from build123d import *

# Parameters (mm, degrees)
SKETCH1_R           = 237
SKETCH1_R_2         = 225
BOSS_EXTRUDE1_DEPTH = 2
SKETCH2_R           = 227
SKETCH2_R_2         = 225
EXTRUDE_THIN1_DEPTH = 50
SKETCH3_R           = 237
SKETCH3_R_2         = 225
EXTRUDE_THIN2_DEPTH = 2


with BuildPart() as part:
    # Sketch1 → Boss-Extrude1 (new body)
    with BuildSketch(Plane(origin=(0, 0, 0), x_dir=(1, 0, 0), z_dir=(0, 1, 0))):
        with Locations(Location((0, 0, 0), (0, 0, 270))):
            Circle(SKETCH1_R)
        with Locations(Location((0, 0, 0), (0, 0, 270))):
            Circle(SKETCH1_R_2, mode=Mode.SUBTRACT)
    extrude(amount=BOSS_EXTRUDE1_DEPTH)

    # Sketch2 → Extrude-Thin1 (add)
    with BuildSketch(Plane(origin=(0, 2, 0), x_dir=(1, 0, 0), z_dir=(0, 1, 0))):
        Circle(SKETCH2_R)
        Circle(SKETCH2_R_2, mode=Mode.SUBTRACT)
    extrude(amount=EXTRUDE_THIN1_DEPTH)

    # Sketch3 → Extrude-Thin2 (add)
    with BuildSketch(Plane(origin=(0, 52, 0), x_dir=(1, 0, 0), z_dir=(0, 1, 0))):
        Circle(SKETCH3_R)
        Circle(SKETCH3_R_2, mode=Mode.SUBTRACT)
    extrude(amount=EXTRUDE_THIN2_DEPTH)


solid = part.part
Input: part model. Units: mm. Frame: model coordinates. A direction names the side the tool comes from. Give positions to 0.01 mm unless a question says otherwise; leave off trailing zeros. Loops run counter-clockwise (first coordinate to the right, second up) from the corner with the lowest first, then second, coordinate; pieces in that order, holes last. Notation, with made-up numbers: (82.25, -32.5) -> (108.25, -32.5) arc R14 ccw to (108.25, -22.5) -> close; hole circle Ø11 at (-25, 48). An arc over 180 degrees is marked (long way). Answer as a JSON object with one key per item and string values. Group by question number.
Item 1: Reachability of faces 1 (the flat face through (210, 54, 87)), 2 (the cylindrical face through (-167.308, 26.65, -153.417)) from +Z, -Z, +X, -X, +Y, -Y: full face, straight path, thin tool, end or side. Return the list, or none.
Item 2: Cut plane B-B, the plane z = -47. Return the cut outline in (x, y), and give its area (3 significant figures).
Item 3: Line query: probe 1 along X at (y, z) = (19, 0); probe 2 along Z at (x, y) = (66.5, 48). Output: solid intervals per line, ascending.
Item 4: Cut plane C-C, the plane y = 7.5. Return the cut outline in (x, z).
Item 5: Pin query (flat end, axial travel): P1, Ø12, axis at x = 128, y = 26.5, coming from the +Z side; P2, Ø1, axis at y = 28, z = -152, coming from the +X side; P3, Ø4, axis at y = 44, z = -22, coming from the -X side. Return the tip coordinate at first contact, or that it passes through.
Checks:
{
 "1": {"face 1": "+Z, -Z, +X, -X, +Y", "face 2": "none"},
 "2": {"outline": "(-232.29, 0) -> (-220.04, 0) -> (-220.04, 54) -> (-232.29, 54) -> (-232.29, 52) -> (-222.08, 52) -> (-222.08, 2) -> (-232.29, 2) -> close; (220.04, 0) -> (232.29, 0) -> (232.29, 2) -> (222.08, 2) -> (222.08, 52) -> (232.29, 52) -> (232.29, 54) -> (220.04, 54) -> close", "area": "303 mm²"},
 "3": {"probe 1": "x = -227 to -225, 225 to 227", "probe 2": "z = -217.04 to -214.95, 214.95 to 217.04"},
 "4": {"outline": "circle Ø454 at (0, 0); hole circle Ø450 at (0, 0)"},
 "5": {"P1": "stops at z = 191.43", "P2": "stops at x = 169.05", "P3": "stops at x = -226.12"}
}
